Read the model definition and answer for the solid it produces. Units are mm, in the model's axes. A direction names the side the tool comes from. Round coordinates to 2 decimals unless told otherwise and drop trailing zeros. Order: outer loops, then holes, each group sorted by start corner. A loop starts at its lowest first (then second) coordinate and runs counter-clockwise, first axis right, second up. Notation, with made-up numbers: (-21.5, 59.5) -> (18.5, 59.5) arc R25 ccw to (18.5, 89.5) -> close; hole circle Ø11 at (56, 38). An arc over 180 degrees is marked (long way). Use a Markdown table: item, result. Add a question column.
1. The mould has two halves that part along X. Classify faces 3 (the face through (-18.655, -0.479, 3.944)), 4 (the face through (-1, -5, 4)), 5 (the face through (-4, 0, 4)), 6 (the face through (-39.43, -4.4, 4.06)): +X half, -X half, draft (parallel to the pull), parting line (faces both ways), or undercut.
2. Section D-D, the plane x = 17.5 is taken. Give the vertices of the cut face in (y, z), then the cut area to 3 significant figures.
3. Consider L1, parallel to Y at x = -17.5, z = 2.75; L2, parallel to Y at x = 7, z = 3.5; L3, parallel to X at y = 2.75, z = 2.5. Determine where each line is inside the solid, lowest interval first. Write a range as [from, to].
4. Section B-B, the plane x = 0 is taken. Give the vertices of the cut face in (y, z).
5. Given pin 1 (3 mm diameter, centred on x = -17.5, y = 0, fed in from -Z); pin 2 (2.5 mm diameter, centred on x = 0, y = 0, fed in from +Z); pin 3 (1 mm diameter, centred on y = -4, z = 6, fed in from -X), each flat-ended and moving along its own axis, determine where each tip first touches the part or whether it passes through.
6. Section A-A, the plane z = 4.75 is taken. Give the number of separate pieces and of enclosed holes in the cut face, then the cut area to 3 significant figures.
7. For faces 1 (the face through (40, 0, 4)), 2 (the face through (9, -3, 4)), determine the directions among +Z, -Z, +X, -X, +Y, -Y from which every point of the face is accessible in a straight line to the end or side of a thin tool.
```python
from build123d import *

# Parameters (mm, degrees)
SKETCH_1_W             = 80
SKETCH_1_H             = 10
EXTRUDE_1_DEPTH        = 8
HOLE_WIZARD_M5_1_D     = 4.2
HOLE_WIZARD_M5_1_DEPTH = 12.4
HOLE_WIZARD_M5_1_TIP   = 1.2618073
HOLE_WIZARD_M3_1_D     = 2.5
HOLE_WIZARD_M3_1_DEPTH = 17.5
HOLE_WIZARD_M3_1_TIP   = 0.751075774
FILLET_1_R             = 2
CUT_EXTRUDE_1_DEPTH    = 36


with BuildPart() as part:
    # 草图1 → 凸台-拉伸1 (new body)
    with BuildSketch(Plane.XY):
        Rectangle(SKETCH_1_W, SKETCH_1_H)
    extrude(amount=EXTRUDE_1_DEPTH)

    # M5 螺纹孔1
    with Locations(Plane.XY.offset(8)):
        with Locations((-35, 0), (0, 0), (35, 0)):
            Hole(HOLE_WIZARD_M5_1_D / 2, depth=HOLE_WIZARD_M5_1_DEPTH)
            with Locations((0, 0, -(HOLE_WIZARD_M5_1_DEPTH + HOLE_WIZARD_M5_1_TIP / 2))):  # 118° drill point
                Cone(0, HOLE_WIZARD_M5_1_D / 2, HOLE_WIZARD_M5_1_TIP, mode=Mode.SUBTRACT)

    # M3 螺纹孔1
    with Locations(Plane.XY.offset(8)):
        with Locations((-17.5, 0), (17.5, 0)):
            Hole(HOLE_WIZARD_M3_1_D / 2, depth=HOLE_WIZARD_M3_1_DEPTH)
            with Locations((0, 0, -(HOLE_WIZARD_M3_1_DEPTH + HOLE_WIZARD_M3_1_TIP / 2))):  # 118° drill point
                Cone(0, HOLE_WIZARD_M3_1_D / 2, HOLE_WIZARD_M3_1_TIP, mode=Mode.SUBTRACT)

    # 圆角1
    fillet_1_edges = [part.edges().sort_by_distance(p)[0] for p in [
        (40, -5, 4),
        (-40, -5, 4),
        (-40, 5, 4),
        (40, 5, 4),
    ]]
    fillet(fillet_1_edges, radius=FILLET_1_R)

    # 草图8 → 切除-拉伸1 (cut)
    with BuildSketch(Plane.XY.offset(8)):
        with BuildLine():
            Line((-28, 3), (-23.5, 3))
            ThreePointArc((-23.5, 3), (-20.5, 0), (-23.5, -3))
            Line((-23.5, -3), (-28, -3))
            ThreePointArc((-28, -3), (-31, 0), (-28, 3))
        make_face()
        with BuildLine():
            Line((-7, 3), (-11.5, 3))
            ThreePointArc((-11.5, 3), (-14.5, 0), (-11.5, -3))
            Line((-11.5, -3), (-7, -3))
            ThreePointArc((-7, -3), (-4, 0), (-7, 3))
        make_face()
        with BuildLine():
            Line((7, 3), (11.5, 3))
            ThreePointArc((11.5, 3), (14.5, 0), (11.5, -3))
            Line((11.5, -3), (7, -3))
            ThreePointArc((7, -3), (4, 0), (7, 3))
        make_face()
        with BuildLine():
            Line((28, 3), (23.5, 3))
            ThreePointArc((23.5, 3), (20.5, 0), (23.5, -3))
            Line((23.5, -3), (28, -3))
            ThreePointArc((28, -3), (31, 0), (28, 3))
        make_face()
    extrude(amount=-CUT_EXTRUDE_1_DEPTH, mode=Mode.SUBTRACT)


solid = part.part
```
Verdict:
| question | item | result |
|---|---|---|
| 1 | face 3 | undercut |
| 1 | face 4 | draft |
| 1 | face 5 | undercut |
| 1 | face 6 | -X half |
| 2 | outline | (-5, 0) -> (-1.25, 0) -> (-1.25, 8) -> (-5, 8) -> close; (1.25, 0) -> (5, 0) -> (5, 8) -> (1.25, 8) -> close |
| 2 | area | 60.0 mm2 |
| 3 | L1 | y = [-5, -1.25], [1.25, 5] |
| 3 | L2 | y = [-5, -3], [3, 5] |
| 3 | L3 | x = [-40, -29.2], [-22.3, -12.7], [-5.8, 5.8], [12.7, 22.3], [29.2, 40] |
| 4 | outline | (-5, 0) -> (-2.1, 0) -> (-2.1, 8) -> (-5, 8) -> close; (2.1, 0) -> (5, 0) -> (5, 8) -> (2.1, 8) -> close |
| 5 | pin 1 | stops at z = 0 |
| 5 | pin 2 | passes through |
| 5 | pin 3 | stops at x = -39.94 |
| 6 | separate pieces | 1 |
| 6 | enclosed holes | 9 |
| 6 | area | 524 mm2 |
| 7 | face 1 | +Z, -Z, +X, +Y, -Y |
| 7 | face 2 | +Z, -Z |
